Can you work these out from the model? Positions are in its coordinate system, mm. A direction names the side the tool comes from. Round coordinates to 2 decimals unless told otherwise and drop trailing zeros. Order: outer loops, then holes, each group sorted by start corner. A loop starts at its lowest first (then second) coordinate and runs counter-clockwise, first axis right, second up. Notation, with made-up numbers: (-7, 81) -> (36, 81) arc R15 cw to (36, 104) -> close; hole circle Ø1 at (45, 29). An arc over 180 degrees is marked (long way). One line per item, written item: value.
```python
from build123d import *

# Parameters (mm, degrees)
SKETCH2_W                    = 40
SKETCH2_H                    = 792
BASE_FLANGE1_DEPTH           = 2
EDGE_FLANGE1_STRIP_W         = 12
EDGE_FLANGE1_STRIP_H         = 2
EDGE_FLANGE1_STRIP_CUT_DEPTH = 792
EDGE_FLANGE1_DEPTH           = 792
M5_CLEARANCE_HOLE1_D         = 5.8
LPATTERN1_COUNT              = 5
LPATTERN1_PITCH              = 193
FILLET1_R                    = 15


# Sheet-metal steps are written as plain solids
with BuildPart() as part:
    # Sketch2 → Base-Flange1 (new body)
    with BuildSketch(Plane.XY):
        Rectangle(SKETCH2_W, SKETCH2_H)
    extrude(amount=-BASE_FLANGE1_DEPTH)

    # Edge-Flange1 strip (across the edge) → Edge-Flange1 strip cut (cut)
    with BuildSketch(Plane(origin=(20, -396, 0), x_dir=(-1, 0, 0), z_dir=(0, 1, 0))):
        with Locations((-2, -1)):
            Rectangle(EDGE_FLANGE1_STRIP_W, EDGE_FLANGE1_STRIP_H)
    extrude(amount=EDGE_FLANGE1_STRIP_CUT_DEPTH, mode=Mode.SUBTRACT)

    # Edge-Flange1 section (across the edge) → Edge-Flange1 (add)
    with BuildSketch(Plane(origin=(20, -396, 0), x_dir=(-1, 0, 0), z_dir=(0, 1, 0))):
        with BuildLine():
            Line((0, 2), (0, 33))
            Line((0, 33), (2, 33))
            Line((2, 33), (2, 2))
            ThreePointArc((2, 2), (2.585786438, 0.585786438), (4, 0))
            Line((4, 0), (4, -2))
            ThreePointArc((4, -2), (1.171572875, -0.828427125), (0, 2))
        make_face()
    extrude(amount=EDGE_FLANGE1_DEPTH)

    # M5 Clearance Hole1 (through all)
    with Locations(Plane.XY):
        with Locations((6.0075, -386)):
            m5_clearance_hole1 = Hole(M5_CLEARANCE_HOLE1_D / 2)

    # LPattern1: M5 Clearance Hole1 ×5
    with Locations(*[(0, i * LPATTERN1_PITCH, 0) for i in range(1, LPATTERN1_COUNT)]):
        add(m5_clearance_hole1, mode=Mode.SUBTRACT)

    # Fillet1
    fillet1_edges = [part.edges().sort_by_distance(p)[0] for p in [
        (19, -396, 33),
        (19, 396, 33),
        (-20, -396, -1),
        (-20, 396, -1),
    ]]
    fillet(fillet1_edges, radius=FILLET1_R)


solid = part.part
```
Q1. I want a section at A-A on y = -182.5. List the corners of the cut face in (x, z) for me, plus the area to 3 significant figures.
Answers below:
outline: (-20, -2) -> (16, -2) arc R4 ccw to (20, 2) -> (20, 33) -> (18, 33) -> (18, 2) arc R2 cw to (16, 0) -> (-20, 0) -> close
area: 143 mm^2
Q2. Please list where these lines run through material, in increasing order: line 1 along X through (y, z) = (-193, -1.55); line 2 along Z through (x, y) = (-12, -275.5); line 3 along X through (y, z) = (210, 19.5).
Answers below:
line 1: -20 to 3.11, 8.91 to 17.84
line 2: -2 to 0
line 3: 18 to 20
Q3. Will these pins go through, and if not, where does the flat tip stop? pin 1 Ø4 at (x, y) = (1, 117.5) entering from +Z; pin 2 Ø12 at (y, z) = (-152.5, 24.5) entering from -X; pin 3 Ø4.5 at (x, y) = (6.01, 386) entering from -Z.
Answers below:
pin 1: z = 0
pin 2: x = 18
pin 3: through
Q4. I want a section at B-B on z = 12. List the corners of the cut face in (x, y) for me, plus the area to 3 significant figures.
Answers below:
outline: (18, -396) -> (20, -396) -> (20, 396) -> (18, 396) -> close
area: 1,580 mm^2
Q5. On a 3-axis mill with a long thin cutter (end or side, diameter ignored), from which of +Z, -Z, +X, -X, +Y, -Y can I reach the whole of each face in a straight line? I mean faces 1 (the face through (18.99, 391.49, 28.72)), 2 (the face through (-2, 6, 0)). Say none if no direction works.
Answers below:
face 1: +Z, +X, -X, +Y
face 2: +Z, -X, +Y, -Y
Q6. I want a section at C-C on x = -13. List the corners of the cut face in (y, z) for me.
Answers below:
outline: (-393.69, -2) -> (393.69, -2) -> (393.69, 0) -> (-393.69, 0) -> close
